Work out the finished part from the listing and answer in its coordinate system (mm). Face numbers are marked on the shaded views. A direction names the side the tool comes from. Coordinates: 2 decimals unless noted, no trailing zeros. Write each loop counter-clockwise with the first axis right and the second up, starting at its lowest first coordinate (ties: lowest second). Pieces come first, ordered by that corner, then holes. Notation, with made-up numbers: (7, 62) - (52, 62) arc R22 ccw to (52, 93) - close; hole circle Ø11 at (-38, -18). An arc over 180 degrees is marked (long way). One line per item, written item: value.
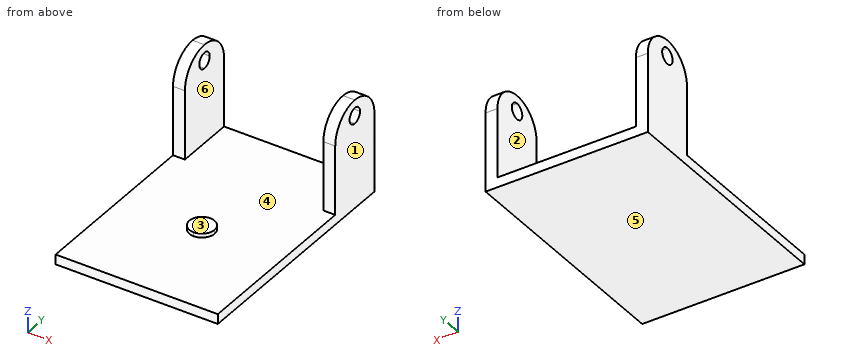
```python
from build123d import *

# Parameters (mm, degrees)
F0_W     = 82
F0_H     = 120
F1_DEPTH = 5
F3_DEPTH = 2
F4_W     = 6
F4_H     = 30
F5_DEPTH = 50
F7_DEPTH = 82.001
F8_R     = 14.99999


# Not quite as in the source:
# - a fillet or chamfer is up to 0.001 mm smaller than in the source, because OpenCascade refuses the exact size


with BuildPart() as f1:
    # F0 (on Top) → F1 (new body)
    with BuildSketch(Plane.XY):
        with Locations((-1.9225833714, 0.167620076)):
            Rectangle(F0_W, F0_H)
    extrude(amount=F1_DEPTH)

    # F2 (on face) → F3 (join)
    with BuildSketch(Plane.XY.offset(5)):
        with BuildLine():
            ThreePointArc((-1.9225833714, -16.2103295776), (2.5873080787, -14.3422713741), (4.4553662822, -9.832379924))
            ThreePointArc((4.4553662822, -9.832379924), (-6.4324748215, -5.3224884739), (-1.9225833714, -16.2103295776))
        make_face()
    extrude(amount=F3_DEPTH)

    # F4 (on face) → F5 (join)
    with BuildSketch(Plane.XY.offset(5)):
        with Locations((-39.9225833714, 45.167620076)):
            Rectangle(F4_W, F4_H)
        with Locations((36.0774166286, 45.167620076)):
            Rectangle(F4_W, F4_H)
    extrude(amount=F5_DEPTH)

    # F6 (on face) → F7 (cut, through all)
    with BuildSketch(Plane.YZ.offset(39.0774166286)):
        with BuildLine():
            Line((45.167620076, 43), (45.167620076, 51))
            ThreePointArc((45.167620076, 51), (41.167620076, 47), (45.167620076, 43))
        make_face()
        with BuildLine():
            ThreePointArc((45.167620076, 43), (47.9960472007, 44.1715728753), (49.167620076, 47))
            ThreePointArc((49.167620076, 47), (47.9960472007, 49.8284271247), (45.167620076, 51))
            Line((45.167620076, 51), (45.167620076, 43))
        make_face()
    extrude(amount=-F7_DEPTH, mode=Mode.SUBTRACT)

    # F8 (radius 15 in the source; OpenCascade refuses exactly that, so slightly less here)
    f8_edges = [f1.edges().sort_by_distance(p)[0] for p in [
        (36.077417, 30.16762, 55),
        (-39.922583, 30.16762, 55),
        (-39.922583, 60.16762, 55),
        (36.077417, 60.16762, 55),
    ]]
    fillet(f8_edges, radius=F8_R)


solid = f1.part
```
Item 1: Determine the mould class of the marked faces 1, 2, 3 and 4 for opening direction X: +X half, -X half, draft (parallel to the pull), parting line (faces both ways), or undercut.
Evaluation:
face 1: +X half
face 2: undercut
face 3: draft
face 4: undercut
Item 2: Section A-A, the plane z = 17 is taken. Determine the outline of the cut face in (x, y), then the cut area to 3 significant figures.
Evaluation:
outline: (-42.92, 30.17) - (-36.92, 30.17) - (-36.92, 60.17) - (-42.92, 60.17) - close; (33.08, 30.17) - (39.08, 30.17) - (39.08, 60.17) - (33.08, 60.17) - close
area: 360 mm2
Item 3: Section C-C, the plane x = -29 is taken. Determine the outline of the cut face in (y, z), then the cut area to 3 significant figures.
Evaluation:
outline: (-59.83, 0) - (60.17, 0) - (60.17, 5) - (-59.83, 5) - close
area: 600 mm2
Item 4: Section B-B, the plane z = 49.5 is taken. Determine the outline of the cut face in (x, y).
Evaluation:
outline: (-42.92, 33.56) - (-36.92, 33.56) - (-36.92, 42.05) - (-42.92, 42.05) - close; (-42.92, 48.29) - (-36.92, 48.29) - (-36.92, 56.78) - (-42.92, 56.78) - close; (33.08, 33.56) - (39.08, 33.56) - (39.08, 42.05) - (33.08, 42.05) - close; (33.08, 48.29) - (39.08, 48.29) - (39.08, 56.78) - (33.08, 56.78) - close
Item 5: Given pin 1 (2 mm diameter, centred on x = 20.5, y = -8, fed in from +Z); pin 2 (3 mm diameter, centred on x = -40.5, z = 16, fed in from -Y); pin 3 (24.5 mm diameter, centred on x = 9.5, y = -12.5, fed in from +Z), each flat-ended and moving along its own axis, determine where each tip first touches the part or whether it passes through.
Evaluation:
pin 1: stops at z = 5
pin 2: stops at y = 30.17
pin 3: stops at z = 7
Item 6: Consider probe 1 along X at (y, z) = (45, 42); probe 2 along Z at (x, y) = (24, -38.5); probe 3 along Y at (x, z) = (-38.5, 8.5). Determine where each line is inside the solid, lowest interval first.
Evaluation:
probe 1: x = -42.92 to -36.92, 33.08 to 39.08
probe 2: z = 0 to 5
probe 3: y = 30.17 to 60.17
Item 7: Section D-D, the plane y = -33 is taken. Determine the outline of the cut face in (x, z), then the cut area to 3 significant figures.
Evaluation:
outline: (-42.92, 0) - (39.08, 0) - (39.08, 5) - (-42.92, 5) - close
area: 410 mm2
Item 8: Which of the six approach directions +Z, -Z, +X, -X, +Y, -Y give full straight-line access (tool end or side, diameter ignored) to the marked faces 5 and 6?
Evaluation:
face 5: -Z, +X, -X, +Y, -Y
face 6: +Z, +Y, -Y
